Input: dimensioned drawing with shaded views. Units: mm. Origin: part minimum x, y, z. A direction names the side the tool comes from. Give positions to 0.01 mm unless a question says otherwise; leave off trailing zeros. Order: outer loops, then holes, each group sorted by start corner. A loop starts at its lowest first (then second) coordinate and runs counter-clockwise, first axis right, second up.
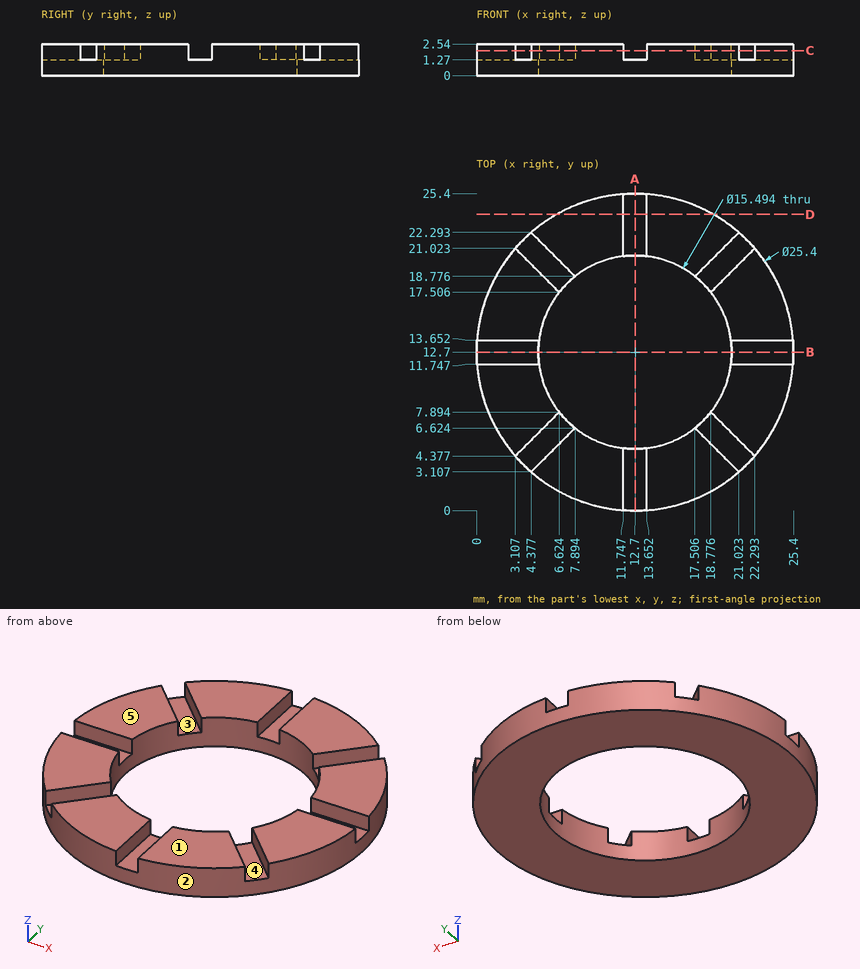
1) Reachability of the marked faces 4 and 5 from +Z, -Z, +X, -X, +Y, -Y: full face, straight path, thin tool, end or side. Return the list, or none.
2) First-contact query: P1, Ø1, axis at y = 19.5, z = 0.5, coming from the +X side; P2, Ø1, axis at x = 12.5, y = 3.5, coming from the +Z side; P3, Ø8, axis at x = 15, y = 12, coming from the +Z side; P4, Ø1, axis at x = 14, z = 1.5, coming from the -Y side. Flat tips, straight axial feed; report the tip coordinate or a pass-through.
3) Pull-direction query (X, two-part tool) for the marked faces 1, 2 and 3; classes: pulls with the +X half, pulls with the -X half, needs draft (parallel to the pull), parting line crosses it, or undercut.
4) Cut plane C-C (z = 2). Count the separate pieces of the cut face and the enclosed holes in it, then the cut area to 3 significant figures.
5) Cut plane A-A (x = 12.7). Return the cut outline in (y, z), then the cut area to 3 significant figures.
6) Cut plane D-D (y = 23.75). Return the cut outline in (x, z).
7) Line query: probe 1 along Y at (x, z) = (12.7, 1); probe 2 along Y at (x, z) = (19.5, 2.4) (1 decimal). Output: solid intervals per line, ascending.
Geometry says:
1. face 4: +Z
1. face 5: +Z, +X, -X, +Y, -Y
2. P1: stops at x = 23.73
2. P2: stops at z = 1.27
2. P3: passes through
2. P4: stops at y = 0.03
3. face 1: needs draft
3. face 2: parting line crosses it
3. face 3: undercut
4. separate pieces: 8
4. enclosed holes: 0
4. area: 245 mm2
5. outline: (0, 0) - (4.95, 0) - (4.95, 1.27) - (0, 1.27) - close; (20.45, 0) - (25.4, 0) - (25.4, 1.27) - (20.45, 1.27) - close
5. area: 12.6 mm2
6. outline: (6.44, 0) - (18.96, 0) - (18.96, 2.54) - (13.65, 2.54) - (13.65, 1.27) - (11.75, 1.27) - (11.75, 2.54) - (6.44, 2.54) - close
7. probe 1: y = 0 to 4.95, 20.45 to 25.4
7. probe 2: y = 2 to 4.6, 7.2 to 9, 16.4 to 18.2, 20.8 to 23.4
